Autodesk Fusion 360 part; units mm, degrees
sketch "Sketch1" plane through (0, 0, 0) normal (0, 0, 1) x (1, 0, 0)
  line L0 (-30, 13) -> (-30, 5) construction
  line L1 (-25, 13) -> (-25, 5) construction
  line L2 (-32, 6) -> (-22, 6) construction
  line L3 (-28.75, 6) -> (-26.25, 6)
  line L4 (-26.2078, 8.4993) -> (-28.7496, 8.5)
  arc A0 (-26.25, 6) -> (-26.2915, 8.4993) centre (-26.25, 7.25) ccw
  arc A1 (-28.7496, 8.5) -> (-28.75, 6) centre (-28.75, 7.25) ccw
  line L5 (-28.7496, 9.75) -> (-26.25, 9.75)
  line L6 (-26.25, 4.75) -> (-28.75, 4.75)
  arc A2 (-26.25, 4.75) -> (-26.25, 9.75) centre (-26.25, 7.25) ccw
  arc A3 (-28.7496, 9.75) -> (-28.75, 4.75) centre (-28.75, 7.25) ccw
  dimension "d1" = 5
  dimension "d2" = 1.25
  dimension "d3" = 1.25
  dimension "d4" = 5
extrude "Extrude1" add sketch "Sketch1" along normal blind 0.2
sketch "Sketch2" plane through (0, 0, 0.2) normal (0, 0, 1) x (-1, 0, 0)
  arc A0 (28.7496, -8.5) -> (28.75, -6) centre (28.75, -7.25) ccw
  line L0 (28.7496, -8.5) -> (26.2915, -8.4993)
  arc A1 (26.25, -6) -> (26.2915, -8.4993) centre (26.25, -7.25) ccw
  line L1 (26.25, -6) -> (28.75, -6)
  arc A2 (26.25, -4.75) -> (26.25, -9.75) centre (26.25, -7.25) ccw
  line L2 (26.25, -9.75) -> (28.7496, -9.75)
  arc A3 (28.7496, -9.75) -> (28.75, -4.75) centre (28.75, -7.25) ccw
  line L3 (28.75, -4.75) -> (26.25, -4.75)
extrude "Extrude2" add sketch "Sketch2" along normal blind 0.5 contours A0 L0 A1 L1 | A2 L2 A3 L3
fillet "Fillet1" radius 0.2 4 edges at (-27.5, 4.75, 0.7) (-23.75, 7.25, 0.7) (-27.4998, 9.75, 0.7) (-31.25, 7.2502, 0.7)
Check sheet for the modelled part. Datum: model origin and axes. Units: mm. Give positions to 0.01 mm unless a question says otherwise; leave off trailing zeros. Write each loop counter-clockwise with the first axis right and the second up, starting at its lowest first coordinate (ties: lowest second). Pieces come first, ordered by that corner, then holes. Notation, with made-up numbers: (-8, 61) -> (0, 61) arc R23 cw to (0, 71) -> close; hole circle Ø5 at (19.25, 45). An arc over 180 degrees is marked (long way). One line per item, written item: value. Start each with the question number.
Item 1: Material ranges on probe 1 along Y at (x, z) = (-28.5, 0.05); probe 2 along Z at (x, y) = (-28.5, 8.25); probe 3 along Y at (x, z) = (-30.25, 0.15), recorded low to high. Write a range as from..to.
Item 2: Section check A-A on y = 7.25. Record the cut outline in (x, z).
Item 3: Draft check along Y on faces 1 (the cylindrical face through (-23.75, 7.3, 0.25)), 2 (the flat face through (-27.6, 5.6, 0)), 3 (the flat face through (-27, 7, 0.2)). Enter one of: +Y half, -Y half, draft (parallel to the pull), parting line (faces both ways), or undercut.
Item 4: Section check B-B on x = -27.25. Record the cut outline in (y, z), then the cut area to 3 significant figures.
Item 5: Gauge pin test, flat ends, axial feed: pin 1 (2 mm diameter, centred on x = -26, y = 6.5, fed in from -Z); pin 2 (0.8 mm diameter, centred on x = -26.5, y = 7, fed in from -Z). Record the tip position at first contact, or that the pin passes through.
Results list:
1. probe 1: 4.75..6, 8.5..9.75
1. probe 2: 0.2..0.7
1. probe 3: 5.25..9.25
2. outline: (-31.25, 0) -> (-30, 0) -> (-30, 0.2) -> (-25, 0.2) -> (-25, 0) -> (-23.75, 0) -> (-23.75, 0.5) arc R0.2 ccw to (-23.95, 0.7) -> (-31.05, 0.7) arc R0.2 ccw to (-31.25, 0.5) -> close
3. face 1: parting line
3. face 2: draft
3. face 3: undercut
4. outline: (4.75, 0) -> (6, 0) -> (6, 0.2) -> (8.5, 0.2) -> (8.5, 0) -> (9.75, 0) -> (9.75, 0.5) arc R0.2 ccw to (9.55, 0.7) -> (4.95, 0.7) arc R0.2 ccw to (4.75, 0.5) -> close
4. area: 2.98 mm²
5. pin 1: z = 0
5. pin 2: z = 0.2
